from build123d import *

# Parameters (mm, degrees)
F1_DEPTH = 4.4958
F3_DEPTH = 4.4968


with BuildPart() as f1:
    # F0 (on Top) → F1 (new body)
    with BuildSketch(Plane.XY):
        Polygon((33.655, 57.15), (-33.655, 57.15), (-33.655, 38.1), (-38.1508, 38.1), (-38.1508, 12.7), (-33.655, 12.7), (-33.655, 0), (-33.655, -12.7), (-38.1508, -12.7), (-38.1508, -38.1), (-33.655, -38.1), (-33.655, -57.15), (33.655, -57.15), (33.655, -38.1), (38.1508, -38.1), (38.1508, -12.7), (33.655, -12.7), (33.655, 0), (33.655, 12.7), (38.1508, 12.7), (38.1508, 38.1), (33.655, 38.1), align=None)
    extrude(amount=F1_DEPTH)

    # F2 (on face) → F3 (cut, through all)
    with BuildSketch(Plane.XY.offset(4.4958)):
        Polygon((25.4, 52.07), (-25.4, 52.07), (-25.4, 45.974), (-9.525, 45.974), (9.525, 45.974), (25.4, 45.974), align=None)
    extrude(amount=-F3_DEPTH, mode=Mode.SUBTRACT)


solid = f1.part
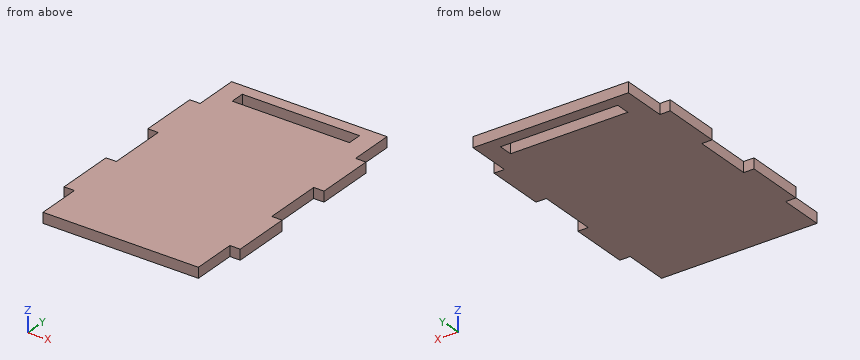
Model file for the job. Use its own axes, mm. Give positions to 0.01 mm unless a question says otherwise; leave off trailing zeros. Loops run counter-clockwise (first coordinate to the right, second up) from the corner with the lowest first, then second, coordinate; pieces in that order, holes last.
1) Wall check: line 1 (Y direction, x = -35, z = 2.05); line 2 (X direction, y = 52, z = 3.7) (3 decimals); line 3 (Y direction, x = 9.5, z = 0.4). Give the ranges that are in metal, low to high.
2) Saw through at B-B (y = 50). Write the cut outline in (x, z) (3 decimals), plus the area to 3 significant figures.
3) Saw through at A-A (z = 1.05). Write the cut outline in (x, y) (3 decimals), plus the area to 3 significant figures.
4) Saw through at C-C (x = 4.5). Write the cut outline in (y, z), plus the area to 3 significant figures.
5) Saw through at D-D (y = -49). Write the cut outline in (x, z) (3 decimals).
6) Flat gauge pins, fed straight in: pin 1 Ø2 at (x, y) = (29, -44.5) entering from -Z; pin 2 Ø1.3 at (x, z) = (36, 2.5) entering from -Y; pin 3 Ø1.3 at (y, z) = (46, 1.5) entering from +X (3 decimals); pin 4 Ø2 at (x, z) = (-36.5, 1.5) entering from +Y. Where does each tip first touch, or does it go through?
Answer block:
1. line 1: y = -38.1 to -12.7, 12.7 to 38.1
1. line 2: x = -33.655 to -25.4, 25.4 to 33.655
1. line 3: y = -57.15 to 45.97, 52.07 to 57.15
2. outline: (-33.655, 0) - (-25.4, 0) - (-25.4, 4.496) - (-33.655, 4.496) - close; (25.4, 0) - (33.655, 0) - (33.655, 4.496) - (25.4, 4.496) - close
2. area: 74.2 mm2
3. outline: (-38.151, -38.1) - (-33.655, -38.1) - (-33.655, -57.15) - (33.655, -57.15) - (33.655, -38.1) - (38.151, -38.1) - (38.151, -12.7) - (33.655, -12.7) - (33.655, 12.7) - (38.151, 12.7) - (38.151, 38.1) - (33.655, 38.1) - (33.655, 57.15) - (-33.655, 57.15) - (-33.655, 38.1) - (-38.151, 38.1) - (-38.151, 12.7) - (-33.655, 12.7) - (-33.655, -12.7) - (-38.151, -12.7) - close; hole (-25.4, 45.974) - (25.4, 45.974) - (25.4, 52.07) - (-25.4, 52.07) - close
3. area: 7,840 mm2
4. outline: (-57.15, 0) - (45.97, 0) - (45.97, 4.5) - (-57.15, 4.5) - close; (52.07, 0) - (57.15, 0) - (57.15, 4.5) - (52.07, 4.5) - close
4. area: 486 mm2
5. outline: (-33.655, 0) - (33.655, 0) - (33.655, 4.496) - (-33.655, 4.496) - close
6. pin 1: stops at z = 0
6. pin 2: stops at y = -38.1
6. pin 3: stops at x = 33.655
6. pin 4: stops at y = 38.1
